Could you check a few things on this model? Use its own coordinates, in mm. Face numbers are marked on the shaded views. A direction names the side the tool comes from. Give positions to 0.01 mm unless a question says otherwise; leave off trailing zeros. Write each loop counter-clockwise with the first axis right and the second up, starting at its lowest first coordinate (ties: lowest second). Pieces come first, ordered by that corner, then holes. Notation, with made-up numbers: M 6,35 L 13,35 A23 cw 13,74 Z; hole C 1.5,33 d6. An arc over 180 degrees is marked long. Answer as a JSON object with one key per item and string values. Group by question number.
```python
from build123d import *

# Parameters (mm, degrees)
SKETCH1_R                = 3.96875
BOSS_EXTRUDE1_DEPTH      = 34.925
BOSS_EXTRUDE1_DEPTH_BACK = 3.175
FILLET1_R                = 3.175
CUT_EXTRUDE1_DEPTH       = 31.1625
CUT_EXTRUDE1_DEPTH_BACK  = 31.1625
SKETCH3_R                = 2.38125
BOSS_EXTRUDE9_DEPTH      = 3.175
MIRROR22_COPY_1_SKETCH_R = 2.38125
MIRROR22_COPY_1_DEPTH    = 3.175


with BuildPart() as part:
    # Sketch1 → Boss-Extrude1 (new body, two sides)
    with BuildSketch(Plane(origin=(0, 0, 0), x_dir=(1, 0, 0), z_dir=(0, 1, 0))) as boss_extrude1_sk:
        Polygon((0, 152.4), (-30.1625, 0), (-30.1625, -15.875), (30.1625, -15.875), (30.1625, 0), align=None)
        with Locations(Location((-18.542, -7.9375, 0), (0, 0, 270))):  # turned: the seam where the file's is
            Circle(SKETCH1_R, mode=Mode.SUBTRACT)
        with Locations(Location((18.542, -7.9375, 0), (0, 0, 270))):  # turned: the seam where the file's is
            Circle(SKETCH1_R, mode=Mode.SUBTRACT)
        Polygon((-26.925913336, 0), (26.925913336, 0), (0, 136.046720015), align=None, mode=Mode.SUBTRACT)
    extrude(amount=BOSS_EXTRUDE1_DEPTH)
    extrude(boss_extrude1_sk.sketch, amount=-BOSS_EXTRUDE1_DEPTH_BACK)

    # Fillet1
    fillet1_edges = [part.edges().sort_by_distance(p)[0] for p in [
        (-26.925913336, 15.875, 0),
        (26.925913336, 15.875, 0),
    ]]
    fillet(fillet1_edges, radius=FILLET1_R)

    # Sketch2 → Cut-Extrude1 (cut, two sides)
    with BuildSketch(Plane(origin=(0, 0, 0), x_dir=(0, 0, -1), z_dir=(1, 0, 0))) as cut_extrude1_sk:
        Polygon((152.4, 15.875), (3.175, 34.925), (152.4, 34.925), align=None)
        Polygon((3.175, -3.175), (152.4, 15.875), (152.4, -3.175), align=None)
    extrude(amount=CUT_EXTRUDE1_DEPTH, mode=Mode.SUBTRACT)
    extrude(cut_extrude1_sk.sketch, amount=-CUT_EXTRUDE1_DEPTH_BACK, mode=Mode.SUBTRACT)

    # Sketch3 → Boss-Extrude9 (add, along a direction that is not the sketch's normal)
    with BuildSketch(Plane(origin=(0, 0, 0), x_dir=(-1, 0, 0), z_dir=(0, -0.99194978, -0.126631887))):
        with BuildLine():
            Line((-16.21869923, 23.183375104), (-24.161406287, 30.114007256))
            Line((-24.161406287, 30.114007256), (-27.516419153, 13.02479135))
            Line((-27.516419153, 13.02479135), (-17.542962116, 16.438061361))
            ThreePointArc((-17.542962116, 16.438061361), (-14.93362632, 19.428436466), (-16.21869923, 23.183375104))
        make_face()
        with Locations((-18.828035026, 20.193)):
            Circle(SKETCH3_R, mode=Mode.SUBTRACT)
        with BuildLine():
            Line((-22.928734085, 36.39279135), (-19.573721219, 53.482007256))
            Line((-19.573721219, 53.482007256), (-11.631014161, 46.551375104))
            ThreePointArc((-11.631014161, 46.551375104), (-10.345941252, 42.796436466), (-12.955277048, 39.806061361))
            Line((-12.955277048, 39.806061361), (-22.928734085, 36.39279135))
        make_face()
        with Locations((-14.240349958, 43.561)):
            Circle(SKETCH3_R, mode=Mode.SUBTRACT)
        with BuildLine():
            Line((-18.341049017, 59.76079135), (-14.986036151, 76.850007256))
            Line((-14.986036151, 76.850007256), (-7.043329093, 69.919375104))
            ThreePointArc((-7.043329093, 69.919375104), (-5.758256184, 66.164436466), (-8.36759198, 63.174061361))
            Line((-8.36759198, 63.174061361), (-18.341049017, 59.76079135))
        make_face()
        with Locations((-9.652664889, 66.929)):
            Circle(SKETCH3_R, mode=Mode.SUBTRACT)
        with BuildLine():
            Line((-13.753363948, 83.12879135), (-10.398351083, 100.218007256))
            Line((-10.398351083, 100.218007256), (-2.455644025, 93.287375104))
            ThreePointArc((-2.455644025, 93.287375104), (-1.170571116, 89.532436466), (-3.779906912, 86.542061361))
            Line((-3.779906912, 86.542061361), (-13.753363948, 83.12879135))
        make_face()
        with Locations((-5.064979821, 90.297)):
            Circle(SKETCH3_R, mode=Mode.SUBTRACT)
    boss_extrude9 = extrude(amount=-BOSS_EXTRUDE9_DEPTH, dir=(0, -1, 0))

    # Mirror21: Boss-Extrude9 across plane
    add(boss_extrude9.mirror(Plane(origin=(0, 0, 0), x_dir=(0, 0, 1), z_dir=(1, 0, 0))))

    # Mirror22: Boss-Extrude9 across plane
    add(boss_extrude9.mirror(Plane.ZX.offset(15.875)))

    # Mirror22 copy 1 sketch → Mirror22 copy 1 (add, along a direction that is not the sketch's normal)
    with BuildSketch(Plane(origin=(0, 31.75, 0), x_dir=(1, 0, 0), z_dir=(0, 0.99194978, -0.126631887))):
        with BuildLine():
            Line((-16.21869923, 23.183375104), (-24.161406287, 30.114007256))
            Line((-24.161406287, 30.114007256), (-27.516419153, 13.02479135))
            Line((-27.516419153, 13.02479135), (-17.542962116, 16.438061361))
            ThreePointArc((-17.542962116, 16.438061361), (-14.93362632, 19.428436466), (-16.21869923, 23.183375104))
        make_face()
        with Locations((-18.828035026, 20.193)):
            Circle(MIRROR22_COPY_1_SKETCH_R, mode=Mode.SUBTRACT)
        with BuildLine():
            Line((-22.928734085, 36.39279135), (-19.573721219, 53.482007256))
            Line((-19.573721219, 53.482007256), (-11.631014161, 46.551375104))
            ThreePointArc((-11.631014161, 46.551375104), (-10.345941252, 42.796436466), (-12.955277048, 39.806061361))
            Line((-12.955277048, 39.806061361), (-22.928734085, 36.39279135))
        make_face()
        with Locations((-14.240349958, 43.561)):
            Circle(MIRROR22_COPY_1_SKETCH_R, mode=Mode.SUBTRACT)
        with BuildLine():
            Line((-18.341049017, 59.76079135), (-14.986036151, 76.850007256))
            Line((-14.986036151, 76.850007256), (-7.043329093, 69.919375104))
            ThreePointArc((-7.043329093, 69.919375104), (-5.758256184, 66.164436466), (-8.36759198, 63.174061361))
            Line((-8.36759198, 63.174061361), (-18.341049017, 59.76079135))
        make_face()
        with Locations((-9.652664889, 66.929)):
            Circle(MIRROR22_COPY_1_SKETCH_R, mode=Mode.SUBTRACT)
        with BuildLine():
            Line((-13.753363948, 83.12879135), (-10.398351083, 100.218007256))
            Line((-10.398351083, 100.218007256), (-2.455644025, 93.287375104))
            ThreePointArc((-2.455644025, 93.287375104), (-1.170571116, 89.532436466), (-3.779906912, 86.542061361))
            Line((-3.779906912, 86.542061361), (-13.753363948, 83.12879135))
        make_face()
        with Locations((-5.064979821, 90.297)):
            Circle(MIRROR22_COPY_1_SKETCH_R, mode=Mode.SUBTRACT)
    extrude(amount=-MIRROR22_COPY_1_DEPTH, dir=(0, 1, 0))


solid = part.part
```
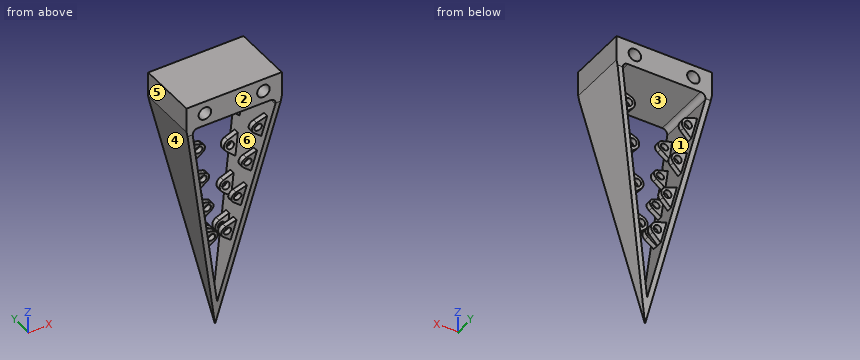
1) I'm going to push flat-ended pins straight in: pin 1 (10 mm diameter, centred on x = 1.5, z = -120, fed in from -Y); pin 2 (10 mm diameter, centred on y = 6.5, z = -23.5, fed in from -X); pin 3 (3 mm diameter, centred on y = 14.5, z = -62, fed in from +X); pin 4 (10.5 mm diameter, centred on x = 18.54, z = 7.94, fed in from -Y) (3 decimals). Where does each tip first touch, or does it pass through?
2) For the marked faces 1, 2 and 3, which set-ups out of +Z, -Z, +X, -X, +Y, -Y let a thin tool reach every point of the face, with its end or its side?
3) Please list where these lines run through material, in increasing order: line 1 along Z through (x, y) = (-4, 32) (3 decimals); line 2 along X through (y, z) = (7.5, -70.5); line 3 along X through (y, z) = (7, -59). Write a range as from..to.
4) If we section it at B-B, the plane z = -72: List the corners of the cut face in (x, y) for me.
5) If we section it at A-A, the plane z = -106: List the corners of the cut face in (x, y) for me.
6) We'd pull the mould along Z, two halves only. Please class the marked faces 4, 5 and 6: released by +Z, released by -Z, zero draft, split by the parting line, or undercut.
Taken from the geometry:
{
 "1": {"pin 1": "y = 11.19", "pin 2": "x = -26.5", "pin 3": "x = 18.19", "pin 4": "y = -3.175"},
 "2": {"face 1": "none", "face 2": "+Z, -Z, +X, -X, -Y", "face 3": "+Y, -Y"},
 "3": {"line 1": "0..15.875", "line 2": "-16.21..-12.97, 12.97..16.21", "line 3": "-18.49..-15.25, 15.25..18.49"},
 "4": {"outline": "M -15.91,5.61 L -12.68,5.61 L -12.68,9.19 L -10.1,9.19 L -10.1,12.37 L -12.68,12.37 L -12.68,19.38 L -10.1,19.38 L -10.1,22.56 L -12.68,22.56 L -12.68,26.14 L -15.91,26.14 Z; M 10.1,9.19 L 12.68,9.19 L 12.68,5.61 L 15.91,5.61 L 15.91,26.14 L 12.68,26.14 L 12.68,22.56 L 10.1,22.56 L 10.1,19.38 L 12.68,19.38 L 12.68,12.37 L 10.1,12.37 Z"},
 "5": {"outline": "M -9.18,9.95 L -5.95,9.95 L -5.95,21.8 L -9.18,21.8 Z; M 5.95,9.95 L 9.18,9.95 L 9.18,21.8 L 5.95,21.8 Z"},
 "6": {"face 4": "released by -Z", "face 5": "zero draft", "face 6": "undercut"}
}
